Here's how the part is built. I have some questions about the finished solid (model axes, mm). A direction names the side the tool comes from. Round coordinates to 2 decimals unless told otherwise and drop trailing zeros. Return JSON: item names as keys, results as strings. Group by question number.
```python
from build123d import *

# Parameters (mm, degrees)
F1_DEPTH = 180


with BuildPart() as f1:
    # F0 (on Top) → F1 (new body)
    with BuildSketch(Plane.XY):
        with BuildLine():
            Line((-3.75, 12.5), (-12, 12.5))
            ThreePointArc((-12, 12.5), (-12.353553, 12.353553), (-12.5, 12))
            Line((-12.5, 12), (-12.5, 3.75))
            ThreePointArc((-12.5, 3.75), (-12.353553, 3.396447), (-12, 3.25))
            Line((-12, 3.25), (-10.87, 3.25))
            ThreePointArc((-10.87, 3.25), (-10.516447, 3.396447), (-10.37, 3.75))
            Line((-10.37, 3.75), (-10.37, 6.845))
            ThreePointArc((-10.37, 6.845), (-10.223553, 7.198553), (-9.87, 7.345))
            Line((-9.87, 7.345), (-9.058244, 7.345))
            ThreePointArc((-9.058244, 7.345), (-8.866903, 7.30694), (-8.704691, 7.198553))
            Line((-8.704691, 7.198553), (-4.526447, 3.020309))
            ThreePointArc((-4.526447, 3.020309), (-4.41806, 2.858097), (-4.38, 2.666756))
            Line((-4.38, 2.666756), (-4.38, 0))
            Line((-4.38, 0), (-4.38, -2.666756))
            ThreePointArc((-4.38, -2.666756), (-4.41806, -2.858097), (-4.526447, -3.020309))
            Line((-4.526447, -3.020309), (-8.704691, -7.198553))
            ThreePointArc((-8.704691, -7.198553), (-8.866903, -7.30694), (-9.058244, -7.345))
            Line((-9.058244, -7.345), (-9.87, -7.345))
            ThreePointArc((-9.87, -7.345), (-10.223553, -7.198553), (-10.37, -6.845))
            Line((-10.37, -6.845), (-10.37, -3.75))
            ThreePointArc((-10.37, -3.75), (-10.516447, -3.396447), (-10.87, -3.25))
            Line((-10.87, -3.25), (-12, -3.25))
            ThreePointArc((-12, -3.25), (-12.353553, -3.396447), (-12.5, -3.75))
            Line((-12.5, -3.75), (-12.5, -12))
            ThreePointArc((-12.5, -12), (-12.353553, -12.353553), (-12, -12.5))
            Line((-12, -12.5), (-3.75, -12.5))
            ThreePointArc((-3.75, -12.5), (-3.396447, -12.353553), (-3.25, -12))
            Line((-3.25, -12), (-3.25, -10.87))
            ThreePointArc((-3.25, -10.87), (-3.396447, -10.516447), (-3.75, -10.37))
            Line((-3.75, -10.37), (-6.845, -10.37))
            ThreePointArc((-6.845, -10.37), (-7.198553, -10.223553), (-7.345, -9.87))
            Line((-7.345, -9.87), (-7.345, -9.058244))
            ThreePointArc((-7.345, -9.058244), (-7.30694, -8.866903), (-7.198553, -8.704691))
            Line((-7.198553, -8.704691), (-3.020309, -4.526447))
            ThreePointArc((-3.020309, -4.526447), (-2.858097, -4.41806), (-2.666756, -4.38))
            Line((-2.666756, -4.38), (0, -4.38))
            Line((0, -4.38), (2.666756, -4.38))
            ThreePointArc((2.666756, -4.38), (2.858097, -4.41806), (3.020309, -4.526447))
            Line((3.020309, -4.526447), (7.198553, -8.704691))
            ThreePointArc((7.198553, -8.704691), (7.30694, -8.866903), (7.345, -9.058244))
            Line((7.345, -9.058244), (7.345, -9.87))
            ThreePointArc((7.345, -9.87), (7.198553, -10.223553), (6.845, -10.37))
            Line((6.845, -10.37), (3.75, -10.37))
            ThreePointArc((3.75, -10.37), (3.396447, -10.516447), (3.25, -10.87))
            Line((3.25, -10.87), (3.25, -12))
            ThreePointArc((3.25, -12), (3.396447, -12.353553), (3.75, -12.5))
            Line((3.75, -12.5), (12, -12.5))
            ThreePointArc((12, -12.5), (12.353553, -12.353553), (12.5, -12))
            Line((12.5, -12), (12.5, -3.75))
            ThreePointArc((12.5, -3.75), (12.353553, -3.396447), (12, -3.25))
            Line((12, -3.25), (10.87, -3.25))
            ThreePointArc((10.87, -3.25), (10.516447, -3.396447), (10.37, -3.75))
            Line((10.37, -3.75), (10.37, -6.845))
            ThreePointArc((10.37, -6.845), (10.223553, -7.198553), (9.87, -7.345))
            Line((9.87, -7.345), (9.058244, -7.345))
            ThreePointArc((9.058244, -7.345), (8.866903, -7.30694), (8.704691, -7.198553))
            Line((8.704691, -7.198553), (4.526447, -3.020309))
            ThreePointArc((4.526447, -3.020309), (4.41806, -2.858097), (4.38, -2.666756))
            Line((4.38, -2.666756), (4.38, 0))
            Line((4.38, 0), (4.38, 2.666756))
            ThreePointArc((4.38, 2.666756), (4.41806, 2.858097), (4.526447, 3.020309))
            Line((4.526447, 3.020309), (8.704691, 7.198553))
            ThreePointArc((8.704691, 7.198553), (8.866903, 7.30694), (9.058244, 7.345))
            Line((9.058244, 7.345), (9.87, 7.345))
            ThreePointArc((9.87, 7.345), (10.223553, 7.198553), (10.37, 6.845))
            Line((10.37, 6.845), (10.37, 3.75))
            ThreePointArc((10.37, 3.75), (10.516447, 3.396447), (10.87, 3.25))
            Line((10.87, 3.25), (12, 3.25))
            ThreePointArc((12, 3.25), (12.353553, 3.396447), (12.5, 3.75))
            Line((12.5, 3.75), (12.5, 12))
            ThreePointArc((12.5, 12), (12.353553, 12.353553), (12, 12.5))
            Line((12, 12.5), (3.75, 12.5))
            ThreePointArc((3.75, 12.5), (3.396447, 12.353553), (3.25, 12))
            Line((3.25, 12), (3.25, 10.87))
            ThreePointArc((3.25, 10.87), (3.396447, 10.516447), (3.75, 10.37))
            Line((3.75, 10.37), (6.845, 10.37))
            ThreePointArc((6.845, 10.37), (7.198553, 10.223553), (7.345, 9.87))
            Line((7.345, 9.87), (7.345, 9.058244))
            ThreePointArc((7.345, 9.058244), (7.30694, 8.866903), (7.198553, 8.704691))
            Line((7.198553, 8.704691), (3.020309, 4.526447))
            ThreePointArc((3.020309, 4.526447), (2.858097, 4.41806), (2.666756, 4.38))
            Line((2.666756, 4.38), (0, 4.38))
            Line((0, 4.38), (-2.666756, 4.38))
            ThreePointArc((-2.666756, 4.38), (-2.858097, 4.41806), (-3.020309, 4.526447))
            Line((-3.020309, 4.526447), (-7.198553, 8.704691))
            ThreePointArc((-7.198553, 8.704691), (-7.30694, 8.866903), (-7.345, 9.058244))
            Line((-7.345, 9.058244), (-7.345, 9.87))
            ThreePointArc((-7.345, 9.87), (-7.198553, 10.223553), (-6.845, 10.37))
            Line((-6.845, 10.37), (-3.75, 10.37))
            ThreePointArc((-3.75, 10.37), (-3.396447, 10.516447), (-3.25, 10.87))
            Line((-3.25, 10.87), (-3.25, 12))
            ThreePointArc((-3.25, 12), (-3.396447, 12.353553), (-3.75, 12.5))
        make_face()
        with BuildLine():
            ThreePointArc((-1.767767, 1.767767), (-0.956709, 2.309699), (0, 2.5))
            ThreePointArc((0, 2.5), (0.956709, 2.309699), (1.767767, 1.767767))
            ThreePointArc((1.767767, 1.767767), (2.309699, 0.956709), (2.5, 0))
            ThreePointArc((2.5, 0), (2.309699, -0.956709), (1.767767, -1.767767))
            ThreePointArc((1.767767, -1.767767), (0.956709, -2.309699), (0, -2.5))
            ThreePointArc((0, -2.5), (-0.956709, -2.309699), (-1.767767, -1.767767))
            ThreePointArc((-1.767767, -1.767767), (-2.309699, -0.956709), (-2.5, 0))
            ThreePointArc((-2.5, 0), (-2.309699, 0.956709), (-1.767767, 1.767767))
        make_face(mode=Mode.SUBTRACT)
    extrude(amount=F1_DEPTH)


solid = f1.part
```
1) I need wall thicknesses on line 1 along Y through (x, z) = (6.75, 103.5); line 2 along Y through (x, z) = (4.75, 94); line 3 along Y through (x, z) = (11.25, 49.5). Which ranges of each line are inside material? Lowest first, please.
2) If we mould it in two halves opening along Y, with no side actions, what happens to faces 6 (the flat face through (12.5, -8, 89)), 7 (the flat face through (-5, 10.37, 89)), 8 (the flat face through (8, -12.5, 89))? For each: released by +Y, released by -Y, zero draft, split by the parting line, or undercut.
3) For faces 1 (the flat face through (4.38, 0, 89)), 2 (the flat face through (0, -4.38, 89)), 3 (the flat face through (-12.5, 8, 89)), 4 (the flat face through (0, 4.38, 89)), 5 (the flat face through (5.08, -6.586, 88.74)), which set-ups out of +Z, -Z, +X, -X, +Y, -Y let a thin tool reach every point of the face, with its end or its side?
4) Will these pins go through, and if not, where does the flat tip stop? pin 1 Ø4 at (y, z) = (0.5, 22) entering from -X; pin 2 Ø6 at (x, y) = (4.5, -8) entering from -Z; pin 3 Ø5 at (y, z) = (1, 26.5) entering from -X; pin 4 Ø2.5 at (x, z) = (0.5, 120.5) entering from -Y.
Results found:
{
 "1": {"line 1": "y = -12.5 to -10.37, -8.26 to -5.24, 5.24 to 8.26, 10.37 to 12.5", "line 2": "y = -12.5 to -10.37, -6.26 to -3.24, 3.24 to 6.26, 10.37 to 12.5", "line 3": "y = -12.5 to -3.25, 3.25 to 12.5"},
 "2": {"face 6": "zero draft", "face 7": "undercut", "face 8": "released by -Y"},
 "3": {"face 1": "+Z, -Z, +X", "face 2": "+Z, -Z, -Y", "face 3": "+Z, -Z, -X, +Y, -Y", "face 4": "+Z, -Z, +Y", "face 5": "+Z, -Z"},
 "4": {"pin 1": "stops at x = -4.38", "pin 2": "stops at z = 0", "pin 3": "stops at x = -12.43", "pin 4": "stops at y = -4.38"}
}
